For this review, take the finished solid that the model builds, in its own axes (mm). A direction names the side the tool comes from. Give positions to 0.01 mm unless a question says otherwise; leave off trailing zeros. Order: outer loops, then holes, each group sorted by start corner. A loop starts at its lowest first (then second) coordinate and runs counter-clockwise, first axis right, second up. Notation, with made-up numbers: (73, 68) - (108, 68) arc R19 cw to (108, 104) - close; hole circle Ø4 at (63, 7.5). An arc over 180 degrees is marked (long way). Answer as a JSON object with one key per item and string values. Group by question number.
from build123d import *

# Parameters (mm, degrees)
SKETCH1_R           = 10
BOSS_EXTRUDE1_DEPTH = 40
FILLET1_R           = 1
FILLET2_R           = 1
SKETCH2_R           = 3
CUT_EXTRUDE1_DEPTH  = 41
CUT_EXTRUDE2_REACH  = 22
SKETCH4_R           = 1


with BuildPart() as part:
    # Sketch1 → Boss-Extrude1 (new body)
    with BuildSketch(Plane(origin=(0, 0, 0), x_dir=(1, 0, 0), z_dir=(0, 1, 0))):
        Circle(SKETCH1_R)
    extrude(amount=BOSS_EXTRUDE1_DEPTH)

    # Fillet1
    fillet1_edges = [part.edges().sort_by_distance(p)[0] for p in [
        (-10, 40, 0),
    ]]
    fillet(fillet1_edges, radius=FILLET1_R)

    # Fillet2
    fillet2_edges = [part.edges().sort_by_distance(p)[0] for p in [
        (-10, 0, 0),
    ]]
    fillet(fillet2_edges, radius=FILLET2_R)

    # Sketch2 → Cut-Extrude1 (cut, through all)
    with BuildSketch(Plane(origin=(0, 40, 0), x_dir=(1, 0, 0), z_dir=(0, 1, 0))):
        Circle(SKETCH2_R)
    extrude(amount=-CUT_EXTRUDE1_DEPTH, mode=Mode.SUBTRACT)

    # Sketch4 → Cut-Extrude2 (cut, up to next)
    with BuildSketch(Plane(origin=(0, 40, 10), x_dir=(1, 0, 0), z_dir=(0, 0, 1)), mode=Mode.PRIVATE) as cut_extrude2_sk1:
        with Locations((0, -4.106598233)):
            Circle(SKETCH4_R)
    cut_extrude2_tool1 = extrude(cut_extrude2_sk1.sketch, amount=-CUT_EXTRUDE2_REACH, mode=Mode.PRIVATE) & part.part
    add(cut_extrude2_tool1.solids().sort_by_distance((0, 35.893402, 10))[0], mode=Mode.SUBTRACT)
    # Sketch4 → Cut-Extrude2 (cut, up to next)
    with BuildSketch(Plane(origin=(0, 40, 10), x_dir=(1, 0, 0), z_dir=(0, 0, 1)), mode=Mode.PRIVATE) as cut_extrude2_sk2:
        with Locations((0, -24.106598233)):
            Circle(SKETCH4_R)
    cut_extrude2_tool2 = extrude(cut_extrude2_sk2.sketch, amount=-CUT_EXTRUDE2_REACH, mode=Mode.PRIVATE) & part.part
    add(cut_extrude2_tool2.solids().sort_by_distance((0, 15.893402, 10))[0], mode=Mode.SUBTRACT)


solid = part.part
1) For pin 1 (1 mm diameter, centred on x = -4.5, y = 16.5, fed in from -Z); pin 2 (5 mm diameter, centred on x = 0, z = 0, fed in from -Y); pin 3 (1.5 mm diameter, centred on y = 16, z = 5, fed in from +X); pin 4 (2.5 mm diameter, centred on x = 0, y = 35.89, fed in from +Z), all flat-tipped, find the tip position at first contact; note any pin that passes through.
2) For faces 1 (the face through (0.461, 15.006, 6.465)), 2 (the face through (0, 40, 4)), list the 3-axis set-ups (+Z, -Z, +X, -X, +Y, -Y) from which the entire face can be reached by the end or side of a thin tool; tool diameter is ignored.
3) Consider section D-D (z = 4.75). Give the number of separate pieces and of enclosed holes in the cut face, plus the area to 3 significant figures.
4) Consider section A-A (z = 0). Give the boundary of the cut face in (x, y), plus the area to 3 significant figures.
5) Consider section B-B (x = 0). Give the boundary of the cut face in (y, z).
6) Consider section C-C (y = 23). Give the boundary of the cut face in (x, z), plus the area to 3 significant figures.
7) For line 1 (Y direction, x = 0, z = 4.5); line 2 (X direction, y = 14, z = -0.25); line 3 (X direction, y = 36.5, z = -2.75), list the stretches that pass through material, from the lowest coordinate up.
8) Mouldability with a two-part tool opening along X and no side actions: class faces 3 (the face through (-2.17, 19.73, 9.76)), 4 (the face through (0, 0, 4)), 5 (the face through (1.61, 20.28, -2.53)) as released by +X, released by -X, zero draft, split by the parting line, or undercut.
Result set:
{
 "1": {"pin 1": "stops at z = -9.17", "pin 2": "passes through", "pin 3": "stops at x = 9.05", "pin 4": "stops at z = 10"},
 "2": {"face 1": "+Z", "face 2": "+Z, -Z, +X, -X, +Y"},
 "3": {"separate pieces": "1", "enclosed holes": "2", "area": "697 mm2"},
 "4": {"outline": "(-10, 1) arc R1 ccw to (-9, 0) - (-3, 0) - (-3, 40) - (-9, 40) arc R1 ccw to (-10, 39) - close; (3, 0) - (9, 0) arc R1 ccw to (10, 1) - (10, 39) arc R1 ccw to (9, 40) - (3, 40) - close", "area": "559 mm2"},
 "5": {"outline": "(0, -9) arc R1 ccw to (1, -10) - (39, -10) arc R1 ccw to (40, -9) - (40, -3) - (0, -3) - close; (0, 3) - (14.89, 3) - (14.89, 10) - (1, 10) arc R1 ccw to (0, 9) - close; (16.89, 3) - (34.89, 3) - (34.89, 10) - (16.89, 10) - close; (36.89, 3) - (40, 3) - (40, 9) arc R1 ccw to (39, 10) - (36.89, 10) - close"},
 "6": {"outline": "circle Ø20 at (0, 0); hole circle Ø6 at (0, 0)", "area": "286 mm2"},
 "7": {"line 1": "y = 0 to 14.89, 16.89 to 34.89, 36.89 to 40", "line 2": "x = -10 to -2.99, 2.99 to 10", "line 3": "x = -9.61 to -1.2, 1.2 to 9.61"},
 "8": {"face 3": "split by the parting line", "face 4": "zero draft", "face 5": "undercut"}
}
